Check sheet for the modelled part. Datum: model origin and axes. Units: mm. A direction names the side the tool comes from. Coordinates: 2 decimals unless noted, no trailing zeros. Loops run counter-clockwise (first coordinate to the right, second up) from the corner with the lowest first, then second, coordinate; pieces in that order, holes last. Notation, with made-up numbers: M 71.5,18.25 L 99.5,18.25 A18 cw 99.5,29.25 Z; hole C 10.5,3 d10. An arc over 180 degrees is marked long. Return JSON: item names as keys, results as strings.
from build123d import *

# Parameters (mm, degrees)
SKETCH_1_W           = 105.6
SKETCH_1_H           = 20
EXTRUDE_1_DEPTH      = 3
SKETCH_10_W          = 105.6
SKETCH_10_H          = 20
SKETCH_10_W_2        = 99.6
SKETCH_10_H_2        = 14
EXTRUDE_2_DEPTH      = 20
SKETCH_11_R          = 2
CUT_EXTRUDE_1_DEPTH  = 110
SKETCH_12_W          = 15
SKETCH_12_H          = 23
EXTRUDE_3_DEPTH      = 105.6
SKETCH_14_W          = 99.6
SKETCH_14_H          = 15
CUT_EXTRUDE_2_DEPTH  = 20
CUT_EXTRUDE_3_DEPTH  = 20
SKETCH_17_R          = 1
EXTRUDE_4_DEPTH      = 15
EXTRUDE_4_DEPTH_BACK = 120.6
SKETCH_19_W          = 99.6
SKETCH_19_H          = 29
CUT_EXTRUDE_4_DEPTH  = 10


with BuildPart() as part:
    # 草图1 → 凸台-拉伸1 (new body)
    with BuildSketch(Plane(origin=(0, 0, 0), x_dir=(1, 0, 0), z_dir=(0, 1, 0))):
        Rectangle(SKETCH_1_W, SKETCH_1_H)
    extrude(amount=EXTRUDE_1_DEPTH)

    # 草图10 → 凸台-拉伸2 (add)
    with BuildSketch(Plane(origin=(0, 3, 0), x_dir=(1, 0, 0), z_dir=(0, 1, 0))):
        Rectangle(SKETCH_10_W, SKETCH_10_H)
        Rectangle(SKETCH_10_W_2, SKETCH_10_H_2, mode=Mode.SUBTRACT)
    extrude(amount=EXTRUDE_2_DEPTH)

    # 草图11 → 切除-拉伸1 (cut)
    with BuildSketch(Plane.ZY.offset(52.8)):
        with Locations((0, 13)):
            Circle(SKETCH_11_R)
    extrude(amount=-CUT_EXTRUDE_1_DEPTH, mode=Mode.SUBTRACT)

    # 草图12 → 凸台-拉伸3 (add)
    with BuildSketch(Plane.ZY.offset(52.8)):
        with Locations((17.5, 11.5)):
            Rectangle(SKETCH_12_W, SKETCH_12_H)
    extrude(amount=-EXTRUDE_3_DEPTH)

    # 草图14 → 切除-拉伸2 (cut)
    with BuildSketch(Plane(origin=(0, 23, 0), x_dir=(1, 0, 0), z_dir=(0, 1, 0))):
        with Locations((0, -14.5)):
            Rectangle(SKETCH_14_W, SKETCH_14_H)
    extrude(amount=-CUT_EXTRUDE_2_DEPTH, mode=Mode.SUBTRACT)

    # 草图16 → 切除-拉伸3 (cut)
    with BuildSketch(Plane.XZ):
        with BuildLine():
            ThreePointArc((-33.5, 7.719862672), (-34.671572875, 10.548289796), (-37.5, 11.719862672))
            Line((-37.5, 11.719862672), (-37.5, 3.719862672))
            ThreePointArc((-37.5, 3.719862672), (-34.671572875, 4.891435547), (-33.5, 7.719862672))
        make_face()
        with BuildLine():
            Line((-37.5, 3.719862672), (-37.5, 11.719862672))
            ThreePointArc((-37.5, 11.719862672), (-41.5, 7.719862672), (-37.5, 3.719862672))
        make_face()
        with BuildLine():
            ThreePointArc((41.5, 7.5), (40.328427125, 10.328427125), (37.5, 11.5))
            Line((37.5, 11.5), (37.5, 3.5))
            ThreePointArc((37.5, 3.5), (40.328427125, 4.671572875), (41.5, 7.5))
        make_face()
        with BuildLine():
            Line((37.5, 3.5), (37.5, 11.5))
            ThreePointArc((37.5, 11.5), (33.5, 7.5), (37.5, 3.5))
        make_face()
    extrude(amount=-CUT_EXTRUDE_3_DEPTH, mode=Mode.SUBTRACT)

    # 草图17 → 凸台-拉伸4 (add, two sides)
    with BuildSketch(Plane.ZY.offset(52.8)) as extrude_4_sk:
        with Locations((10, 12)):
            Circle(SKETCH_17_R)
    extrude(amount=EXTRUDE_4_DEPTH)
    extrude(extrude_4_sk.sketch, amount=-EXTRUDE_4_DEPTH_BACK)

    # 草图19 → 切除-拉伸4 (cut)
    with BuildSketch(Plane(origin=(0, 3, 0), x_dir=(1, 0, 0), z_dir=(0, 1, 0))):
        with Locations((0, -7.5)):
            Rectangle(SKETCH_19_W, SKETCH_19_H)
    extrude(amount=CUT_EXTRUDE_4_DEPTH, mode=Mode.SUBTRACT)


solid = part.part
1) Scan lines: line 1 along X through (y, z) = (8, 19); line 2 along Z through (x, y) = (51.85, 13); line 3 along Y through (x, z) = (-51, 0). Record each from-to range of solid material in increasing order. Write a range as [from, to].
Answers:
{"line 1": "[-52.8, -49.8], [49.8, 52.8]", "line 2": "[-10, -2], [2, 25]", "line 3": "[0, 11], [15, 23]"}
2) Section check B-B on y = 9.75. Record the cut outline in (x, z).
Answers:
{"outline": "M -52.8,-10 L 52.8,-10 L 52.8,25 L -52.8,25 Z; hole M -49.8,-7 L 49.8,-7 L 49.8,22 L -49.8,22 Z"}
3) Section check A-A on z = 0. Record the cut outline in (x, y), then the cut area to 3 significant figures.
Answers:
{"outline": "M -52.8,0 L 52.8,0 L 52.8,11 L 49.8,11 L 49.8,3 L -49.8,3 L -49.8,11 L -52.8,11 Z; M -52.8,15 L -49.8,15 L -49.8,23 L -52.8,23 Z; M 49.8,15 L 52.8,15 L 52.8,23 L 49.8,23 Z", "area": "413 mm²"}
4) Section check C-C on x = -27. Record the cut outline in (y, z).
Answers:
{"outline": "M 0,-10 L 23,-10 L 23,-7 L 3,-7 L 3,22 L 23,22 L 23,25 L 0,25 Z"}
5) Draft check along Z on faces 3 (the face through (0, 23, 23)), 4 (the face through (-1, 11, 25)), 5 (the face through (49.8, 13, 8)), 6 (the face through (-49.8, 13, 8)). Enter one of: +Z half, -Z half, draft (parallel to the pull), parting line (faces both ways), or undercut.
Answers:
{"face 3": "draft", "face 4": "+Z half", "face 5": "undercut", "face 6": "undercut"}
6) Go/stop test with flat-tipped pins: pin 1 Ø11.5 at (y, z) = (12.5, 0.5) entering from +X; pin 2 Ø4 at (y, z) = (12.5, 13) entering from -X; pin 3 Ø2.5 at (y, z) = (13, 0) entering from -X; pin 4 Ø12 at (x, z) = (31.5, 5.5) entering from +Y. Record where each tip stops, or that it passes through.
Answers:
{"pin 1": "x = 52.8", "pin 2": "x = -52.8", "pin 3": "through", "pin 4": "y = 3"}
7) Set-up check for faces 1 (the face through (-1, 13, 22)), 2 (the face through (-51, 15, 0)): record each of +Z, -Z, +X, -X, +Y, -Y from which the full face is reachable in a straight line by a thin tool's end or side.
Answers:
{"face 1": "+Y", "face 2": "+X, -X"}
8) Section check D-D on z = 19. Record the cut outline in (x, y).
Answers:
{"outline": "M -52.8,0 L 52.8,0 L 52.8,23 L 49.8,23 L 49.8,3 L -49.8,3 L -49.8,23 L -52.8,23 Z"}
